from build123d import *

# Parameters (mm, degrees)
SKETCH1_W           = 76.2
SKETCH1_H           = 38.1
BOSS_EXTRUDE1_DEPTH = 1.75
FILLET1_R           = 1
SKETCH2_R           = 5
BOSS_EXTRUDE2_DEPTH = 30


with BuildPart() as part:
    # Sketch1 → Boss-Extrude1 (new body)
    with BuildSketch(Plane.XY):
        Rectangle(SKETCH1_W, SKETCH1_H)
    extrude(amount=BOSS_EXTRUDE1_DEPTH)

    # Fillet1
    fillet1_edges = [part.edges().sort_by_distance(p)[0] for p in [
        (38.1, -19.05, 0.875),
        (-38.1, -19.05, 0.875),
        (-38.1, 19.05, 0.875),
        (38.1, 19.05, 0.875),
    ]]
    fillet(fillet1_edges, radius=FILLET1_R)

    # Sketch2 → Boss-Extrude2 (add)
    with BuildSketch(Plane.XY.offset(1.75)):
        with Locations((13.1, 2.95)):
            Circle(SKETCH2_R)
    extrude(amount=-BOSS_EXTRUDE2_DEPTH)


solid = part.part
For this review, take the finished solid that the model builds, in its own axes (mm). A direction names the side the tool comes from. Coordinates: 2 decimals unless noted, no trailing zeros. Loops run counter-clockwise (first coordinate to the right, second up) from the corner with the lowest first, then second, coordinate; pieces in that order, holes last. Notation, with made-up numbers: (-14.75, 60) - (17.25, 60) arc R31 cw to (17.25, 90) - close; hole circle Ø9 at (68.25, 54.5). An arc over 180 degrees is marked (long way). Return JSON: item names as keys, results as strings.
Item 1: Take a section at B-B (x = 13.1). Give the boundary of the cut face in (y, z), then the cut area to 3 significant figures.
Determined:
{"outline": "(-19.05, 0) - (-2.05, 0) - (-2.05, -28.25) - (7.95, -28.25) - (7.95, 0) - (19.05, 0) - (19.05, 1.75) - (-19.05, 1.75) - close", "area": "349 mm2"}
Item 2: Mouldability with a two-part tool opening along X and no side actions: class faces 3 (the flat face through (38.1, 0, 1)), 4 (the flat face through (-1, 0, 0)), 5 (the flat face through (-38.1, 0, 1)) as pulls with the +X half, pulls with the -X half, needs draft (parallel to the pull), parting line crosses it, or undercut.
Determined:
{"face 3": "pulls with the +X half", "face 4": "needs draft", "face 5": "pulls with the -X half"}
Item 3: For faces 1 (the cylindrical face through (17.719, 1.035, -13.927)), 2 (the flat face through (13, 3, -28.25)), list the 3-axis set-ups (+Z, -Z, +X, -X, +Y, -Y) from which the entire face can be reached by the end or side of a thin tool; tool diameter is ignored.
Determined:
{"face 1": "-Z", "face 2": "-Z, +X, -X, +Y, -Y"}
Item 4: Take a section at A-A (y = 2.95). Give the boundary of the cut face in (x, z).
Determined:
{"outline": "(-38.1, 0) - (8.1, 0) - (8.1, -28.25) - (18.1, -28.25) - (18.1, 0) - (38.1, 0) - (38.1, 1.75) - (-38.1, 1.75) - close"}
Item 5: Take a section at C-C (z = -7.5). Give the boundary of the cut face in (x, y).
Determined:
{"outline": "circle Ø10 at (13.1, 2.95)"}
Item 6: For line 1 (Z direction, x = -34, y = -8); line 2 (X direction, y = -1.5, z = -4); line 3 (Y direction, x = 16.5, z = -7.75), list the stretches that pass through material, from the lowest coordinate up.
Determined:
{"line 1": "z = 0 to 1.75", "line 2": "x = 10.82 to 15.38", "line 3": "y = -0.72 to 6.62"}
Item 7: Insertion check: pin 1 (1 mm diameter, centred on x = -10, y = 9.5, fed in from -Z); pin 2 (2 mm diameter, centred on x = 6.5, z = -23.5, fed in from -Y). Each pin has a flat end and moves straight along its axis. Give the tip position at first contact, or say it passes through.
Determined:
{"pin 1": "stops at z = 0", "pin 2": "passes through"}
Item 8: Take a section at D-D (y = -4.5). Give the boundary of the cut face in (x, z), then the cut area to 3 significant figures.
Determined:
{"outline": "(-38.1, 0) - (38.1, 0) - (38.1, 1.75) - (-38.1, 1.75) - close", "area": "133 mm2"}
